Geometry check sheet. Reference: drawing and pictorial views, mm from the part's lowest x, y, z. Coordinates: 2 decimals unless noted, no trailing zeros. Loops run counter-clockwise (first coordinate to the right, second up) from the corner with the lowest first, then second, coordinate; pieces in that order, holes last. Notation, with made-up numbers: (42.25, 55.25) - (72.25, 55.25) arc R22 cw to (72.25, 81.25) - close; hole circle Ø7 at (31.5, -1). An arc over 180 degrees is marked (long way). Use a Markdown table: item, result. Add a question column.
1) Sectioned sample at A-A, the plane y = 971.55. Enter the section's corners in (x, z) (3 decimals), then the cut area to 3 significant figures.
2) Thickness scan on line 1 (X direction, y = 1021, z = 16); line 2 (Y direction, x = 292, z = 11.75); line 3 (Y direction, x = 262, z = 13.5). Record the ranges inside material, lowest first.
3) Sectioned sample at B-B, the plane z = 9.5. Enter the section's corners in (x, y) (3 decimals), then the cut area to 3 significant figures.
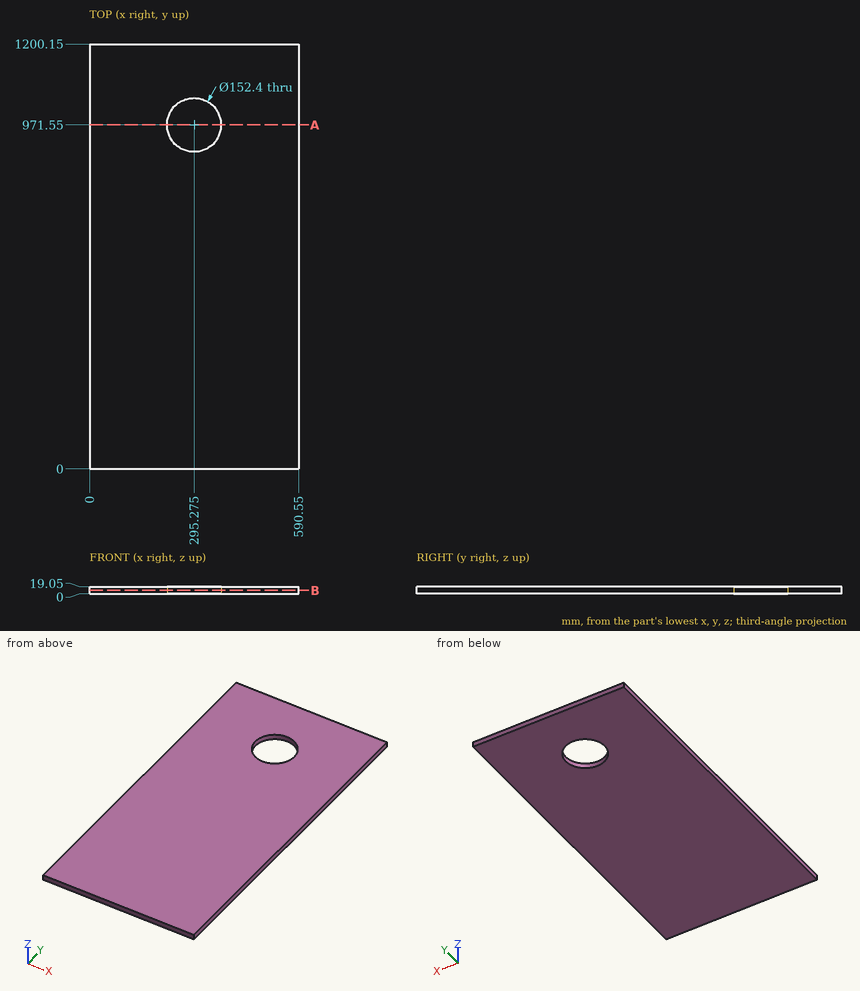
Solved:
| question | item | result |
|---|---|---|
| 1 | outline | (0, 0) - (219.075, 0) - (219.075, 19.05) - (0, 19.05) - close; (371.475, 0) - (590.55, 0) - (590.55, 19.05) - (371.475, 19.05) - close |
| 1 | area | 8,350 mm2 |
| 2 | line 1 | x = 0 to 237.3, 353.25 to 590.55 |
| 2 | line 2 | y = 0 to 895.42, 1047.68 to 1200.15 |
| 2 | line 3 | y = 0 to 903, 1040.1 to 1200.15 |
| 3 | outline | (0, 0) - (590.55, 0) - (590.55, 1200.15) - (0, 1200.15) - close; hole circle Ø152.4 at (295.275, 971.55) |
| 3 | area | 691,000 mm2 |
